from build123d import *

# Parameters (mm, degrees)
EXTRUDE_1_DEPTH          = 2.5
REVOLVE_1_ANGLE          = 70
EXTRUDE_2_DEPTH          = 18.25
EXTRUDE_2_DEPTH_BACK     = 18.25
SKETCH_4_R               = 2.5
SKETCH_4_R_2             = 1
CUT_EXTRUDE_1_DEPTH      = 16.5
CUT_EXTRUDE_1_DEPTH_BACK = 16.5
SKETCH_7_R               = 2.5
SKETCH_7_R_2             = 1
CUT_EXTRUDE_2_DEPTH      = 100
CUT_EXTRUDE_2_DEPTH_BACK = 100
SKETCH_8_R               = 1
SKETCH_9_R               = 1
EXTRUDE_3_DEPTH          = 5
SKETCH_12_R              = 1
CUT_EXTRUDE_3_DEPTH      = 5
EXTRUDE_4_DEPTH          = 2.5
CUT_EXTRUDE_4_DEPTH      = 2.5


with BuildPart() as part:
    # Sketch 1 → Extrude 1 (new body)
    with BuildSketch(Plane.XY):
        with BuildLine():
            Line((-18.25, 0), (-16.5, 0))
            ThreePointArc((-16.5, 0), (0, -16.5), (16.5, 0))
            Line((16.5, 0), (18.25, 0))
            ThreePointArc((18.25, 0), (0, -18.25), (-18.25, 0))
        make_face()
    extrude(amount=EXTRUDE_1_DEPTH)

    # Sketch 2 → Revolve 1 (revolve)
    with BuildSketch(Plane(origin=(0, 0, 0), x_dir=(-1, 0, 0), z_dir=(0, 0, -1))):
        with BuildLine():
            Line((-17.375, 0), (-16.5, 0))
            ThreePointArc((-16.5, 0), (0, -16.5), (16.5, 0))
            Line((16.5, 0), (17.375, 0))
            Line((17.375, 0), (18.25, 0))
            ThreePointArc((18.25, 0), (0, -18.25), (-18.25, 0))
            Line((-18.25, 0), (-17.375, 0))
        make_face()
    revolve(axis=Axis((16.5, 0, 0), (1, 0, 0)), revolution_arc=REVOLVE_1_ANGLE)

    # Sketch 4 → Extrude 2 (add, two sides: drawn at the far end of the back side and taken through both)
    with BuildSketch(Plane(origin=(0, 0, 0), x_dir=(0, 0, -1), z_dir=(1, 0, 0)).offset(-EXTRUDE_2_DEPTH_BACK)):
        with Locations(Location((0, 0, 0), (0, 0, 340))):
            Circle(SKETCH_4_R)
        with Locations(Location((0, 0, 0), (0, 0, 340))):
            Circle(SKETCH_4_R_2, mode=Mode.SUBTRACT)
    extrude(amount=EXTRUDE_2_DEPTH + EXTRUDE_2_DEPTH_BACK)

    # Sketch 7 → Cut-Extrude 1 (cut, two sides: drawn at the far end of the back side and taken through both)
    with BuildSketch(Plane(origin=(0, 0, 0), x_dir=(0, 0, -1), z_dir=(1, 0, 0)).offset(-CUT_EXTRUDE_1_DEPTH_BACK)):
        Circle(SKETCH_7_R)
        Circle(SKETCH_7_R_2, mode=Mode.SUBTRACT)
    extrude(amount=CUT_EXTRUDE_1_DEPTH + CUT_EXTRUDE_1_DEPTH_BACK, mode=Mode.SUBTRACT)

    # Sketch 8 → Cut-Extrude 2 (cut, two sides: drawn at the far end of the back side and taken through both)
    with BuildSketch(Plane(origin=(0, 0, 0), x_dir=(0, 0, -1), z_dir=(1, 0, 0)).offset(-CUT_EXTRUDE_2_DEPTH_BACK)):
        Circle(SKETCH_8_R)
    extrude(amount=CUT_EXTRUDE_2_DEPTH + CUT_EXTRUDE_2_DEPTH_BACK, mode=Mode.SUBTRACT)

    # Sketch 9 → Extrude 3 (add)
    with BuildSketch(Plane.ZY.offset(18.25)):
        with BuildLine():
            Line((1, 0), (2.5, 0))
            Line((2.5, 0), (2.5, -9))
            Line((2.5, -9), (-2.5, -9))
            Line((-2.5, -9), (-2.5, 0))
            Line((-2.5, 0), (-1, 0))
            ThreePointArc((-1, 0), (0, -1), (1, 0))
        make_face()
        with Locations((0, -7)):
            Circle(SKETCH_9_R, mode=Mode.SUBTRACT)
    extrude(amount=-EXTRUDE_3_DEPTH)

    # Sketch 12 → Cut-Extrude 3 (cut)
    with BuildSketch(Plane.ZY.offset(18.25)):
        with Locations((0, -7)):
            Circle(SKETCH_12_R)
    extrude(amount=-CUT_EXTRUDE_3_DEPTH, mode=Mode.SUBTRACT)

    # Sketch 13 → Cut-Revolve 1 (revolve, cut)
    with BuildSketch(Plane.XY):
        with BuildLine():
            Line((16.5, 0), (-16.5, 0))
            ThreePointArc((-16.5, 0), (0, -16.5), (16.5, 0))
        make_face()
    revolve(axis=Axis((16.5, 0, 0), (-1, 0, 0)), mode=Mode.SUBTRACT)

    # Sketch 14 → Extrude 4 (add)
    with BuildSketch(Plane.XY):
        with BuildLine():
            Line((16.5, -1), (19.945657674, -1.473343123))
            ThreePointArc((19.945657674, -1.473343123), (4.12178771, -19.570663404), (-17.657116061, -9.392883071))
            Line((-17.657116061, -9.392883071), (-13.750126888, -9.175184497))
            ThreePointArc((-13.750126888, -9.175184497), (4.31263967, -15.957792425), (16.5, -1))
        make_face()
    extrude(amount=EXTRUDE_4_DEPTH)

    # Sketch 15 → Cut-Extrude 4 (cut)
    with BuildSketch(Plane(origin=(0, 0, 0), x_dir=(-1, 0, 0), z_dir=(0, 0, -1))):
        Polygon((-19.945657674, -1.473343123), (-18.25, -1.240404168), (-18.25, -11.043121242), (-22.78736169, -5.639500824), align=None)
    extrude(amount=-CUT_EXTRUDE_4_DEPTH, mode=Mode.SUBTRACT)


solid = part.part
Design review of the part built by this model. Coordinates are the model's own, in mm. A direction names the side the tool comes from. Round coordinates to 2 decimals unless told otherwise and drop trailing zeros. Order: outer loops, then holes, each group sorted by start corner. A loop starts at its lowest first (then second) coordinate and runs counter-clockwise, first axis right, second up.
1) Consider section A-A (y = -5). State the section outline as (x, z) points.
The answers:
outline: (-18.25, -2.5) - (-17.37, -2.5) arc R17.55 ccw to (-10.92, -13.74) - (-7.65, -13.74) arc R15.72 cw to (-15.52, 2.5) - (-18.25, 2.5) - close; (7.65, -13.74) - (10.92, -13.74) arc R17.55 ccw to (17.55, 0) - (18.25, 0) - (18.25, 2.5) - (15.72, 2.5) - (15.72, 0) arc R15.72 cw to start
2) Consider section C-C (y = -11). State the section outline as (x, z) points.
The answers:
outline: (-16.7, 0) - (-14.56, 0) arc R14.56 ccw to (14.56, 0) - (16.7, 0) - (16.7, 2.5) - (12.3, 2.5) - (12.3, 0) arc R12.3 cw to (-12.3, 0) - (-12.3, 2.5) - (-16.7, 2.5) - close
3) Machinability: for faces 5 (the flat face through (1.71, -18.34, 0)), 6 (the flat face through (-16.5, 1.3, 0)), 7 (the cylindrical face through (16.453, -1.596, 0.875)), 8 (the cylindrical face through (-16, -8, 0)), which of the approach directions +Z, -Z, +X, -X, +Y, -Y give a long, thin tool a straight path to every point of the face, cutting with its end or side? Answer none if there is none.
The answers:
face 5: -Z, -Y
face 6: +Z, -Z, +Y
face 7: +Y
face 8: -X
4) For L1, parallel to Z at x = 17.3, y = 0; L2, parallel to X at y = -4.5, z = -3; L3, parallel to X at y = -14.5, z = -3.75, list the stretches that pass through material, from the lowest coordinate up.
The answers:
L1: z = -2.5 to -1, 1 to 2.5
L2: x = -17.43 to -15.59, 15.59 to 17.43
L3: x = -10.43 to -6.92, 6.92 to 10.43
5) Consider section B-B (x = -9.5). State the section outline as (y, z) points, plus the area to 3 significant figures.
The answers:
outline: (-17.6, 0) - (-15.58, 0) arc R15.58 ccw to (-5.33, -14.64) - (-4.61, -12.68) arc R13.49 cw to (-13.49, 0) - (-13.49, 2.5) - (-17.6, 2.5) - close
area: 47.4 mm2
6) Clearance check with flat-ended pins moving along their axes: pin 1 Ø8 at (x, z) = (6, -11) entering from -Y; pin 2 Ø3 at (y, z) = (0, 0) entering from +X; pin 3 Ø3 at (x, z) = (-17, -1) entering from -Y; pin 4 Ø3 at (x, y) = (-17, -5) entering from -Z. State where each tip first meets the part, or that it passes through.
The answers:
pin 1: stops at y = -16.13
pin 2: stops at x = 18.25
pin 3: stops at y = -12.16
pin 4: stops at z = -8.36
7) Draft analysis for pull direction Y (two halves, no side actions). For faces 1 (the flat face through (-16.7, -9.34, 1.23)), 2 (the flat face through (-18.25, -4, 0)), 3 (the cylindrical face through (0.986, -19.976, 1.232)), 4 (the cylindrical face through (-17, 0, -1)), state which applies: released by +Y, released by -Y, zero draft, split by the parting line, or undercut.
The answers:
face 1: undercut
face 2: zero draft
face 3: released by -Y
face 4: undercut
